Study the drawing (mm; zero at the part's minimum x, y, z) and answer. Round coordinates to 2 decimals unless told otherwise and drop trailing zeros. Loops run counter-clockwise (first coordinate to the right, second up) from the corner with the lowest first, then second, coordinate; pieces in that order, holes last. Notation, with made-up numbers: (-9, 58) -> (40, 58) arc R11 ccw to (40, 72) -> close; hole circle Ø10 at (30, -13). An arc over 180 degrees is marked (long way). Use one line per item in the form item = value.
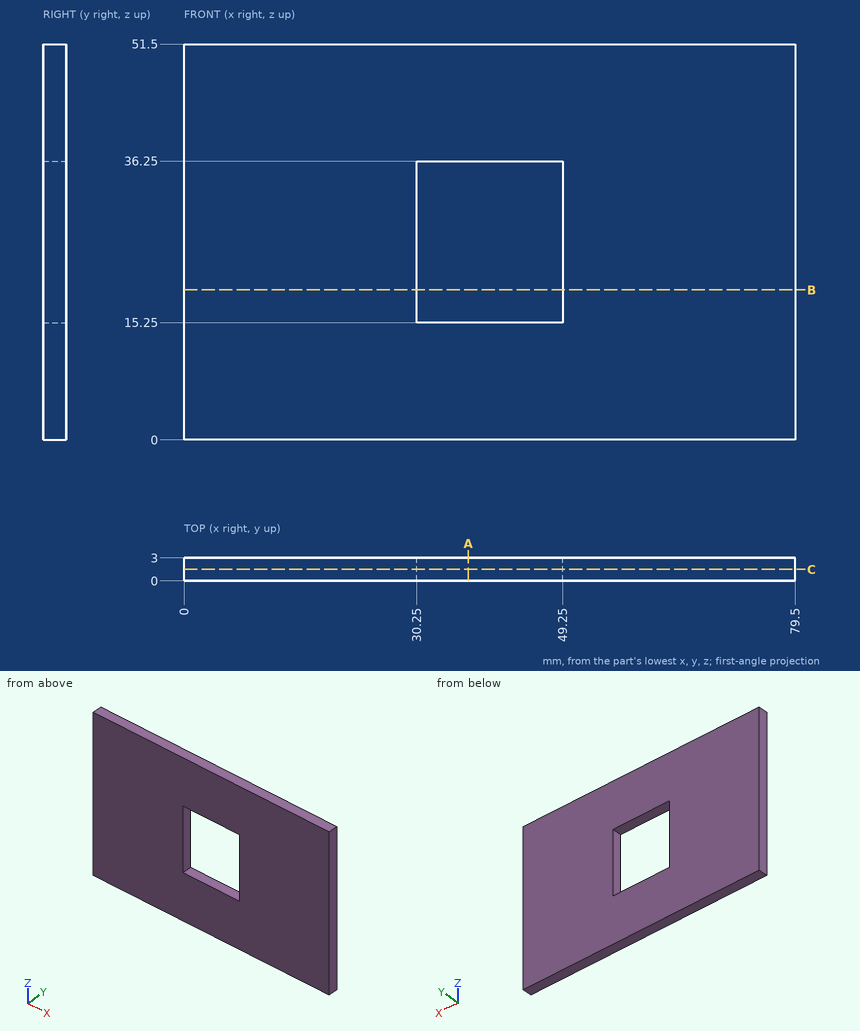
(1) Find section A-A, the plane x = 37. Write down the section's boundary in (y, z).
Completed:
outline = (0, 0) -> (3, 0) -> (3, 15.25) -> (0, 15.25) -> close; (0, 36.25) -> (3, 36.25) -> (3, 51.5) -> (0, 51.5) -> close
(2) Find section B-B, the plane z = 19.5. Write down the section's boundary in (x, y), then the cut area to 4 significant figures.
Completed:
outline = (0, 0) -> (30.25, 0) -> (30.25, 3) -> (0, 3) -> close; (49.25, 0) -> (79.5, 0) -> (79.5, 3) -> (49.25, 3) -> close
area = 181.5 mm2
(3) Find section C-C, the plane y = 1.5. Write down the section's boundary in (x, z), then the cut area to 3 significant figures.
Completed:
outline = (0, 0) -> (79.5, 0) -> (79.5, 51.5) -> (0, 51.5) -> close; hole (30.25, 15.25) -> (49.25, 15.25) -> (49.25, 36.25) -> (30.25, 36.25) -> close
area = 3,700 mm2
(4) Consider L1, parallel to Z at x = 44, y = 1; L2, parallel to X at y = 1.4, z = 36. Determine where each line is inside the solid, lowest interval first.
Completed:
L1 = 0 to 15.25, 36.25 to 51.5
L2 = 0 to 30.25, 49.25 to 79.5
